Check sheet for the modelled part. Datum: model origin and axes. Units: mm. Coordinates: 2 decimals unless noted, no trailing zeros. Loops run counter-clockwise (first coordinate to the right, second up) from the corner with the lowest first, then second, coordinate; pieces in that order, holes last.
```python
from build123d import *

# Parameters (mm, degrees)
F0_W     = 1500
F0_H     = 700
F1_DEPTH = 22
F2_W     = 18.85
F2_H     = 12
F3_DEPTH = 370
F5_D     = 6


with BuildPart() as f1:
    # F0 (on Top) → F1 (new body)
    with BuildSketch(Plane.XY):
        Rectangle(F0_W, F0_H)
        with BuildLine():
            Line((185, -20), (320, -20))
            Line((320, -20), (320, -270))
            Line((320, -270), (-20, -270))
            Line((-20, -270), (-20, -20))
            Line((-20, -20), (115, -20))
            ThreePointArc((115, -20), (150, 15), (185, -20))
        make_face(mode=Mode.SUBTRACT)
    extrude(amount=F1_DEPTH)

    # F2 (on face) → F3 (cut)
    with BuildSketch(Plane.XZ.offset(350)):
        with Locations((-56.046478, 16)):
            Rectangle(F2_W, F2_H)
        with Locations((356.046478, 16)):
            Rectangle(F2_W, F2_H)
    extrude(amount=-F3_DEPTH, mode=Mode.SUBTRACT)

    # F5 (through all)
    with Locations(Plane.XY.offset(22)):
        with Locations((-650, -250), (-550, -250), (-450, -250), (-650, -150), (-550, -150), (-450, -150), (-350, -150), (-250, -150), (-150, -150), (-150, -250), (-350, -250), (-250, -250), (-650, -50), (-650, 50), (-650, 150), (-650, 250), (-550, 250), (-550, 150), (-550, 50), (-550, -50), (-450, -50), (-450, 50), (-450, 150), (-450, 250), (-350, 250), (-250, 250), (-150, 250), (-350, 150), (-350, 50), (-350, -50), (-250, 50), (-250, 150), (-150, 50), (-250, -50), (-150, -50), (-150, 150)):
            Hole(F5_D / 2)


solid = f1.part
```
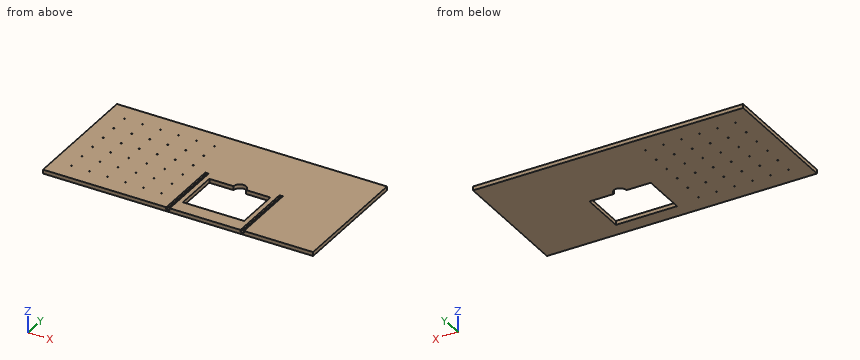
1) Section check C-C on z = 15. Give the number of separate pieces and of enclosed holes in the cut face, plus the area to 3 significant figures.
Answer sheet:
separate pieces: 1
enclosed holes: 37
area: 948,000 mm2
2) Section check B-B on y = -84.5. Enter the section's corners in (x, z).
Answer sheet:
outline: (-750, 0) - (-20, 0) - (-20, 22) - (-46.62, 22) - (-46.62, 10) - (-65.47, 10) - (-65.47, 22) - (-750, 22) - close; (320, 0) - (750, 0) - (750, 22) - (365.47, 22) - (365.47, 10) - (346.62, 10) - (346.62, 22) - (320, 22) - close
3) Section check A-A on x = 150. Enter the section's corners in (y, z).
Answer sheet:
outline: (-350, 0) - (-270, 0) - (-270, 22) - (-350, 22) - close; (15, 0) - (350, 0) - (350, 22) - (15, 22) - close
4) Scan lines: line 1 (X direction, y = -91, z = 19); line 2 (Y direction, x = 24.5, z = 5); line 3 (X direction, y = -244.5, z = 1.25). Record each from-to range of solid material in increasing order.
Answer sheet:
line 1: x = -750 to -65.47, -46.62 to -20, 320 to 346.62, 365.47 to 750
line 2: y = -350 to -270, -20 to 350
line 3: x = -750 to -20, 320 to 750
